Geometry check sheet. Reference: the model listing, model coordinates, mm. Round coordinates to 2 decimals unless told otherwise and drop trailing zeros. Order: outer loops, then holes, each group sorted by start corner. A loop starts at its lowest first (then second) coordinate and runs counter-clockwise, first axis right, second up. Notation, with made-up numbers: (69.5, 16.5) - (99.5, 16.5) arc R17 ccw to (99.5, 41.5) - close; hole circle Ø4 at (64, 41). An arc over 180 degrees is marked (long way). Answer as CSV lines item,"result". Start each with the question number.
```python
from build123d import *

# Parameters (mm, degrees)
F0_R     = 1.5
F1_DEPTH = 1


with BuildPart() as f1:
    # F0 (on Front) → F1 (new body)
    with BuildSketch(Plane.XZ):
        with BuildLine():
            ThreePointArc((39.5, -4.5), (35, 0), (39.5, 4.5))
            Line((39.5, 4.5), (-39.5, 4.5))
            ThreePointArc((-39.5, 4.5), (-36.318019, 3.181981), (-35, 0))
            ThreePointArc((-35, 0), (-36.318019, -3.181981), (-39.5, -4.5))
            Line((-39.5, -4.5), (39.5, -4.5))
        make_face()
        Circle(F0_R, mode=Mode.SUBTRACT)
        with BuildLine():
            ThreePointArc((44, 0), (42.681981, 3.181981), (39.5, 4.5))
            ThreePointArc((39.5, 4.5), (35, 0), (39.5, -4.5))
            ThreePointArc((39.5, -4.5), (42.681981, -3.181981), (44, 0))
        make_face()
        with Locations((39.5, 0)):
            Circle(F0_R, mode=Mode.SUBTRACT)
        with BuildLine():
            ThreePointArc((-35, 0), (-36.318019, 3.181981), (-39.5, 4.5))
            ThreePointArc((-39.5, 4.5), (-44, 0), (-39.5, -4.5))
            ThreePointArc((-39.5, -4.5), (-36.318019, -3.181981), (-35, 0))
        make_face()
        with Locations((-39.5, 0)):
            Circle(F0_R, mode=Mode.SUBTRACT)
    extrude(amount=F1_DEPTH)


solid = f1.part
```
1. Draft check along Z on faces 1 (the face through (-44, -0.5, 0.1)), 2 (the face through (-1.5, -0.49, 0.07)), 3 (the face through (-1, -1, 2)). Enter one of: released by +Z, released by -Z, zero draft, split by the parting line, or undercut.
2. Section check C-C on z = 3.5. Record the boundary of the cut face in (x, y), plus the area to 3 significant figures.
3. Section check A-A on x = 0. Record the boundary of the cut face in (y, z).
4. Thickness scan on probe 1 along Z at (x, y) = (39.5, -0.7); probe 2 along X at (y, z) = (-0.25, 0.75); probe 3 along Z at (x, y) = (38.5, -0.1). Record the ranges inside material, lowest first.
5. Go/stop test with a flat-tipped pin: pin 1 Ø2.5 at (x, z) = (0, 0) entering from -Y. Record where the tip stops, or that it passes through.
Numbers:
1,face 1,"split by the parting line"
1,face 2,"undercut"
1,face 3,"zero draft"
2,outline,"(-42.33, -1) - (42.33, -1) - (42.33, 0) - (-42.33, 0) - close"
2,area,"84.7 mm2"
3,outline,"(-1, -4.5) - (0, -4.5) - (0, -1.5) - (-1, -1.5) - close; (-1, 1.5) - (0, 1.5) - (0, 4.5) - (-1, 4.5) - close"
4,probe 1,"z = -4.5 to -1.5, 1.5 to 4.5"
4,probe 2,"x = -43.94 to -40.8, -38.2 to -1.3, 1.3 to 38.2, 40.8 to 43.94"
4,probe 3,"z = -4.5 to -1.12, 1.12 to 4.5"
5,pin 1,"passes through"
